Read the model definition and answer for the solid it produces. Units are mm, in the model's axes. A direction names the side the tool comes from. Coordinates: 2 decimals unless noted, no trailing zeros. Write each loop counter-clockwise with the first axis right and the second up, starting at its lowest first coordinate (ties: lowest second). Pieces come first, ordered by that corner, then holes.
(1) Section A-A on x = 24 is taken. Write down the section's boundary in (y, z).
(2) The mould has two halves that part along X. Classify faces 1 (the flat face through (127.7, 0, -10)), 2 (the cylindrical face through (157.944, 1.521, -10.032)), 3 (the cylindrical face through (200.39, 1.52, -9.77)): +X half, -X half, draft (parallel to the pull), parting line (faces both ways), or undercut.
(3) Section B-B on z = -9.9 is taken. State how many separate pieces and enclosed holes the cut face has, then the cut area to 3 significant figures.
(4) Which of the six approach directions +Z, -Z, +X, -X, +Y, -Y give full straight-line access (tool end or side, diameter ignored) to faces 4 (the cylindrical face through (128.1, 1.5, -9.8)), 5 (the flat face through (127.7, 3, -10))?
(5) Given pin 1 (0.9 mm diameter, centred on x = 107, y = 1.5, fed in from +Z); pin 2 (1.5 mm diameter, centred on y = 1.5, z = -10.5, fed in from -X), each flat-ended and moving along its own axis, determine where each tip first touches the part or whether it passes through.
(6) Find the intervals of material crossed by probe 1 along Z at (x, y) = (213, 1.8); probe 2 along Z at (x, y) = (49, 2), in increasing order.
from build123d import *

# Parameters (mm, degrees)
SKETCH1_W           = 259
SKETCH1_H           = 19.8
BOSS_EXTRUDE1_DEPTH = 3
SKETCH2_W           = 3
SKETCH2_H           = 11.8
CUT_EXTRUDE1_DEPTH  = 3
CUT_EXTRUDE2_DEPTH  = 3


with BuildPart() as part:
    # Sketch1 → Boss-Extrude1 (new body)
    with BuildSketch(Plane(origin=(0, 0, 0), x_dir=(1, 0, 0), z_dir=(0, 1, 0))):
        with Locations((129.5, 9.9)):
            Rectangle(SKETCH1_W, SKETCH1_H)
    extrude(amount=BOSS_EXTRUDE1_DEPTH)

    # Sketch2 → Cut-Extrude1 (cut)
    with BuildSketch(Plane(origin=(0, 3, 0), x_dir=(1, 0, 0), z_dir=(0, 1, 0))):
        with Locations((1.5, 9.9)):
            Rectangle(SKETCH2_W, SKETCH2_H)
        with Locations((81.5, 9.9)):
            Rectangle(SKETCH2_W, SKETCH2_H)
        with Locations((241.78, 9.9)):
            Rectangle(SKETCH2_W, SKETCH2_H)
    extrude(amount=-CUT_EXTRUDE1_DEPTH, mode=Mode.SUBTRACT)

    # Sketch3 → Cut-Extrude2 (cut)
    with BuildSketch(Plane(origin=(0, 3, 0), x_dir=(1, 0, 0), z_dir=(0, 1, 0))):
        with BuildLine():
            Line((15.291475512, 15.9), (32.057683526, 15.9))
            ThreePointArc((32.057683526, 15.9), (38.057683526, 9.9), (32.057683526, 3.9))
            Line((32.057683526, 3.9), (15.291475512, 3.9))
            ThreePointArc((15.291475512, 3.9), (9.291475512, 9.9), (15.291475512, 15.9))
        make_face()
        with BuildLine():
            Line((97.499979326, 15.9), (117.51125986, 15.9))
            ThreePointArc((117.51125986, 15.9), (123.51125986, 9.9), (117.51125986, 3.9))
            Line((117.51125986, 3.9), (97.499979326, 3.9))
            ThreePointArc((97.499979326, 3.9), (91.499979326, 9.9), (97.499979326, 15.9))
        make_face()
        with BuildLine():
            Line((134.097186069, 15.9), (151.945084923, 15.9))
            ThreePointArc((151.945084923, 15.9), (157.945084923, 9.9), (151.945084923, 3.9))
            Line((151.945084923, 3.9), (134.097186069, 3.9))
            ThreePointArc((134.097186069, 3.9), (128.097186069, 9.9), (134.097186069, 15.9))
        make_face()
        with BuildLine():
            Line((50.266145994, 15.9), (66.491508589, 15.9))
            ThreePointArc((66.491508589, 15.9), (72.491508589, 9.9), (66.491508589, 3.9))
            Line((66.491508589, 3.9), (50.266145994, 3.9))
            ThreePointArc((50.266145994, 3.9), (44.266145994, 9.9), (50.266145994, 15.9))
        make_face()
        with BuildLine():
            Line((168.170447518, 15.9), (188.362009859, 15.9))
            ThreePointArc((188.362009859, 15.9), (194.362009859, 9.9), (188.362009859, 3.9))
            Line((188.362009859, 3.9), (168.170447518, 3.9))
            ThreePointArc((168.170447518, 3.9), (162.170447518, 9.9), (168.170447518, 15.9))
        make_face()
        with BuildLine():
            Line((206.39019052, 15.9), (225.680343827, 15.9))
            ThreePointArc((225.680343827, 15.9), (231.680343827, 9.9), (225.680343827, 3.9))
            Line((225.680343827, 3.9), (206.39019052, 3.9))
            ThreePointArc((206.39019052, 3.9), (200.39019052, 9.9), (206.39019052, 15.9))
        make_face()
    extrude(amount=-CUT_EXTRUDE2_DEPTH, mode=Mode.SUBTRACT)


solid = part.part
Response:
1. outline: (0, -19.8) - (3, -19.8) - (3, -15.9) - (0, -15.9) - close; (0, -3.9) - (3, -3.9) - (3, 0) - (0, 0) - close
2. face 1: draft
2. face 2: undercut
2. face 3: undercut
3. separate pieces: 9
3. enclosed holes: 0
3. area: 203 mm2
4. face 4: +Y, -Y
4. face 5: +Z, -Z, +X, -X, +Y
5. pin 1: stops at z = 0
5. pin 2: stops at x = 3
6. probe 1: z = -19.8 to -15.9, -3.9 to 0
6. probe 2: z = -19.8 to -15.76, -4.04 to 0
